For this review, take the finished solid that the model builds, in its own axes (mm). A direction names the side the tool comes from. Round coordinates to 2 decimals unless told otherwise and drop trailing zeros. Loops run counter-clockwise (first coordinate to the right, second up) from the corner with the lowest first, then second, coordinate; pieces in that order, holes last. Notation, with made-up numbers: (41.25, -3) -> (69.25, -3) arc R14 ccw to (69.25, 1) -> close; hole circle Ø1 at (25, 19). An arc over 180 degrees is marked (long way). Use one line per item in the form item = value. Start each with the question number.
from build123d import *

# Parameters (mm, degrees)
BOSS_EXTRUDE1_DEPTH     = 40
BOSS_EXTRUDE2_DEPTH     = 3
EXTRUDE_THIN1_DEPTH     = 108
CUT_EXTRUDE1_DEPTH      = 124.020323524
CUT_EXTRUDE1_DEPTH_BACK = 12
CHAMFER1_SIZE           = 10
SKETCH5_R               = 2.25
CUT_EXTRUDE2_DEPTH      = 3


with BuildPart() as part:
    # Sketch1 → Boss-Extrude1 (new body)
    with BuildSketch(Plane(origin=(0, 0, 0), x_dir=(1, 0, 0), z_dir=(0, 1, 0))):
        Polygon((-54, 0), (-54, -50), (54, -50), (54, 0), (57, 0), (79, 0), (79, -3), (57, -3), (57, -53), (-57, -53), (-57, -3), (-79, -3), (-79, 0), (-57, 0), align=None)
    extrude(amount=BOSS_EXTRUDE1_DEPTH)

    # Sketch2 → Boss-Extrude2 (add)
    with BuildSketch(Plane.ZY.offset(57)):
        Polygon((53, 40), (15, 78), (0, 78), (0, 40), align=None)
    boss_extrude2 = extrude(amount=-BOSS_EXTRUDE2_DEPTH)

    # Mirror1: Boss-Extrude2 across plane
    add(boss_extrude2.mirror(Plane(origin=(0, 0, 0), x_dir=(0, 0, 1), z_dir=(1, 0, 0))))

    # Sketch3 → Extrude-Thin1 (add)
    with BuildSketch(Plane.ZY.offset(-54)):
        Polygon((0, 78), (15, 78), (53, 40), (50.878679656, 37.878679656), (13.757359313, 75), (0, 75), align=None)
    extrude(amount=EXTRUDE_THIN1_DEPTH)

    # Sketch4 → Cut-Extrude1 (cut, two sides: drawn at the far end of the back side and taken through both)
    with BuildSketch(Plane(origin=(0, 78, 0), x_dir=(1, 0, 0), z_dir=(0, 1, 0)).offset(-CUT_EXTRUDE1_DEPTH_BACK)):
        Polygon((-42, 274.196896272), (-42, 0), (-42, -5), (-32, -15), (32, -15), (42, -5), (42, 0), (42, 274.196896272), (42, 822.590688817), (-42, 822.590688817), align=None)
    extrude(amount=CUT_EXTRUDE1_DEPTH + CUT_EXTRUDE1_DEPTH_BACK, mode=Mode.SUBTRACT)

    # Chamfer1
    chamfer1_edges = [part.edges().sort_by_distance(p)[0] for p in [
        (-79, 40, 1.5),
        (79, 0, 1.5),
        (-79, 0, 1.5),
        (79, 40, 1.5),
    ]]
    chamfer(chamfer1_edges, length=CHAMFER1_SIZE)

    # Sketch5 → Cut-Extrude2 (cut)
    with BuildSketch(Plane.XY.offset(3)):
        with Locations((-72, 20)):
            Circle(SKETCH5_R)
    cut_extrude2 = extrude(amount=-CUT_EXTRUDE2_DEPTH, mode=Mode.SUBTRACT)

    # Mirror2: Cut-Extrude2 across plane
    add(cut_extrude2.mirror(Plane(origin=(0, 0, 0), x_dir=(0, 0, 1), z_dir=(1, 0, 0))), mode=Mode.SUBTRACT)


solid = part.part
Item 1: Take a section at B-B on y = 20. Give the boundary of the cut face in (x, z), plus the area to 3 significant figures.
Item 2: Take a section at A-A on x = 72. Give the boundary of the cut face in (y, z).
Item 3: For P1, Ø4, axis at x = -48, y = 27.5, coming from the -Z side; P2, Ø15, axis at y = 43, z = 18.5, coming from the -X side; P3, Ø7, axis at x = 45, z = 8.5, coming from the -Y side, all flat-tipped, find the tip position at first contact; note any pin that passes through.
Item 4: Wall thickness on line 1 (X direction, y = 15, z = 42.5); line 2 (Y direction, x = 72, z = 0.6); line 3 (Z direction, x = 69, y = 23.5): over which ranges is each line inside the solid? List them lowest first.
Item 5: Take a section at D-D on x = 23.5. Give the boundary of the cut face in (y, z).
Item 6: Take a section at C-C on y = 33.5. Give the boundary of the cut face in (x, z), plus the area to 3 significant figures.
Item 7: Draft analysis for pull direction X (two halves, no side actions). For faces 1 (the flat face through (1, 59, 34)), 2 (the flat face through (0, 76, 15)), 3 (the flat face through (74, 5, 1)), 4 (the flat face through (54, 30, 25)), state which applies: +X half, -X half, draft (parallel to the pull), parting line (faces both ways), or undercut.
Item 8: Machinability: for faces 5 (the flat face through (-37, 76, 10)), 6 (the flat face through (68, 20, 3)), 7 (the flat face through (-63, 40, 1)), 8 (the flat face through (46, 75, 9)), 9 (the flat face through (-68, 20, 3)), which of the approach directions +Z, -Z, +X, -X, +Y, -Y give a long, thin tool a straight path to every point of the face, cutting with its end or side? Answer none if there is none.
Results:
q1.outline = (-79, 0) -> (-74.25, 0) -> (-74.25, 3) -> (-79, 3) -> close; (-69.75, 0) -> (-54, 0) -> (-54, 50) -> (54, 50) -> (54, 0) -> (69.75, 0) -> (69.75, 3) -> (57, 3) -> (57, 53) -> (-57, 53) -> (-57, 3) -> (-69.75, 3) -> close; (74.25, 0) -> (79, 0) -> (79, 3) -> (74.25, 3) -> close
q1.area = 747 mm2
q2.outline = (3, 0) -> (17.75, 0) -> (17.75, 3) -> (3, 3) -> close; (22.25, 0) -> (37, 0) -> (37, 3) -> (22.25, 3) -> close
q3.P1 = 50
q3.P2 = -57
q3.P3 = 75
q4.line_1 = -57 to -54, 54 to 57
q4.line_2 = 3 to 17.75, 22.25 to 37
q4.line_3 = 0 to 3
q5.outline = (0, 50) -> (38.76, 50) -> (73.76, 15) -> (78, 15) -> (40, 53) -> (0, 53) -> close
q6.outline = (-75.5, 0) -> (-54, 0) -> (-54, 50) -> (54, 50) -> (54, 0) -> (75.5, 0) -> (75.5, 3) -> (57, 3) -> (57, 53) -> (-57, 53) -> (-57, 3) -> (-75.5, 3) -> close
q6.area = 753 mm2
q7.face_1 = draft
q7.face_2 = undercut
q7.face_3 = +X half
q7.face_4 = undercut
q8.face_5 = -Z, +Y, -Y
q8.face_6 = +Z, +X, +Y, -Y
q8.face_7 = +Z, -Z, -X, +Y
q8.face_8 = -Z, -Y
q8.face_9 = +Z, -X, +Y, -Y
